Source: CAD feature listing. Evaluate the final solid. Frame: model axes, mm. Face numbers are marked on the shaded views. Coordinates: 2 decimals unless noted, no trailing zeros. Order: outer loops, then holes, each group sorted by start corner. A loop starts at its lowest first (then second) coordinate and runs counter-clockwise, first axis right, second up.
Item 1: Section A-A on y = 5. Return the cut outline in (x, z), then the cut area to 3 significant figures.
Item 2: Section C-C on x = -5. Return the cut outline in (y, z).
Item 3: Ray query, line 1 (X direction, y = 0.25, z = -4); line 2 (Y direction, x = -12.3, z = -4); line 3 (Z direction, x = 5, y = 0.25). Return the intervals inside material, ascending.
Item 4: Mould query, pull axis X, two halves, no side actions, for the marked faces 1, 2 and 3. Classes: released by +X, released by -X, zero draft, split by the parting line, or undercut.
Item 5: Section D-D on z = -1.25. Return the cut outline in (x, y).
Item 6: Section B-B on z = -4. Return the cut outline in (x, y), then the cut area to 3 significant figures.
Item 7: Contact query for flat-ended pins moving along their axis: P1, Ø4, axis at y = 15, z = -4, coming from the -X side; P2, Ø3, axis at y = 10, z = -2.5, coming from the +X side; P3, Ø1, axis at x = -2, z = -6.5, coming from the +Y side. Output: stop coordinate, or through.
from build123d import *

# Parameters (mm, degrees)
BOSS_EXTRUDE1_DEPTH = 0.7
SKETCH3_W           = 0.7
SKETCH3_H           = 8
BOSS_EXTRUDE3_DEPTH = 20
SKETCH4_R           = 2.15
CUT_EXTRUDE1_DEPTH  = 34.42887973


with BuildPart() as part:
    # Sketch1 → Boss-Extrude1 (new body)
    with BuildSketch(Plane(origin=(0, 0, 0), x_dir=(1, 0, 0), z_dir=(0, 1, 0))):
        with BuildLine():
            Line((0, 0), (0, 4))
            Line((0, 4), (-3.5, 4))
            ThreePointArc((-3.5, 4), (-5, 2.5), (-6.5, 4))
            Line((-6.5, 4), (-12.5, 4))
            Line((-12.5, 4), (-12.5, 0))
            Line((-12.5, 0), (0, 0))
        make_face()
        with BuildLine():
            Line((12.5, 4), (6.5, 4))
            ThreePointArc((6.5, 4), (5, 2.5), (3.5, 4))
            Line((3.5, 4), (0, 4))
            Line((0, 4), (0, 0))
            Line((0, 0), (12.5, 0))
            Line((12.5, 0), (12.5, 4))
        make_face()
        with BuildLine():
            ThreePointArc((3.5, 4), (5, 5.5), (6.5, 4))
            Line((6.5, 4), (12.5, 4))
            Line((12.5, 4), (12.5, 8))
            Line((12.5, 8), (0, 8))
            Line((0, 8), (0, 4))
            Line((0, 4), (3.5, 4))
        make_face()
        with BuildLine():
            Line((-3.5, 4), (0, 4))
            Line((0, 4), (0, 8))
            Line((0, 8), (-12.5, 8))
            Line((-12.5, 8), (-12.5, 4))
            Line((-12.5, 4), (-6.5, 4))
            ThreePointArc((-6.5, 4), (-5, 5.5), (-3.5, 4))
        make_face()
    extrude(amount=BOSS_EXTRUDE1_DEPTH)

    # Sketch3 → Boss-Extrude3 (add)
    with BuildSketch(Plane(origin=(0, 0.7, 0), x_dir=(1, 0, 0), z_dir=(0, 1, 0))):
        with Locations((-12.15, 4)):
            Rectangle(SKETCH3_W, SKETCH3_H)
    extrude(amount=BOSS_EXTRUDE3_DEPTH)

    # Sketch4 → Cut-Extrude1 (cut, through all)
    with BuildSketch(Plane.ZY.offset(12.5)):
        with Locations((-4, 5)):
            Circle(SKETCH4_R)
        with Locations((-4, 15)):
            Circle(SKETCH4_R)
    extrude(amount=-CUT_EXTRUDE1_DEPTH, mode=Mode.SUBTRACT)


solid = part.part
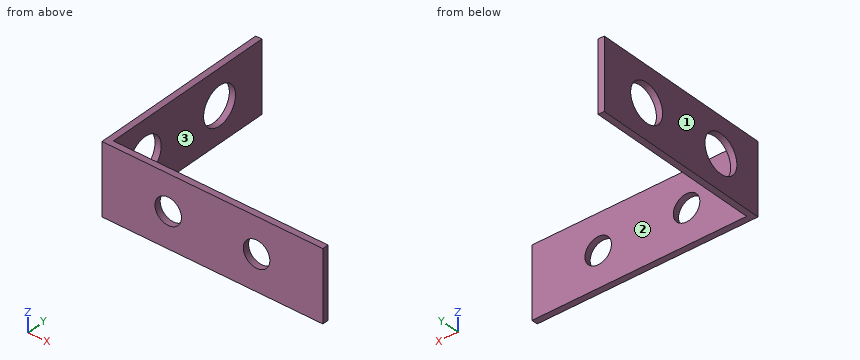
Answer list:
1. outline: (-12.5, -8) - (-11.8, -8) - (-11.8, -6.15) - (-12.5, -6.15) - close; (-12.5, -1.85) - (-11.8, -1.85) - (-11.8, 0) - (-12.5, 0) - close
1. area: 2.59 mm2
2. outline: (0, -8) - (0.7, -8) - (0.7, -5.5) - (0, -5.5) - close; (0, -2.5) - (0.7, -2.5) - (0.7, 0) - (0, 0) - close
3. line 1: x = -12.5 to -6.5, -3.5 to 3.5, 6.5 to 12.5
3. line 2: y = 0 to 2.85, 7.15 to 12.85, 17.15 to 20.7
3. line 3: z = -8 to -5.5, -2.5 to 0
4. face 1: released by -X
4. face 2: zero draft
4. face 3: released by +X
5. outline: (-12.5, 0) - (12.5, 0) - (12.5, 0.7) - (-11.8, 0.7) - (-11.8, 20.7) - (-12.5, 20.7) - close
6. outline: (-12.5, 0) - (-6.5, 0) - (-6.5, 0.7) - (-11.8, 0.7) - (-11.8, 2.85) - (-12.5, 2.85) - close; (-12.5, 7.15) - (-11.8, 7.15) - (-11.8, 12.85) - (-12.5, 12.85) - close; (-12.5, 17.15) - (-11.8, 17.15) - (-11.8, 20.7) - (-12.5, 20.7) - close; (-3.5, 0) - (3.5, 0) - (3.5, 0.7) - (-3.5, 0.7) - close; (6.5, 0) - (12.5, 0) - (12.5, 0.7) - (6.5, 0.7) - close
6. area: 21.3 mm2
7. P1: passes through
7. P2: stops at x = -11.8
7. P3: stops at y = 0.7
